Build history of the part. All positions in model axes, mm. A direction names the side the tool comes from. Give positions to 0.01 mm unless a question says otherwise; leave off trailing zeros. Write each loop counter-clockwise with the first axis right and the second up, starting at its lowest first coordinate (ties: lowest second). Pieces come first, ordered by that corner, then holes.
from build123d import *

# Parameters (mm, degrees)
SKETCH2_W           = 10
SKETCH2_H           = 10
BOSS_EXTRUDE1_DEPTH = 1.6
SKETCH4_W           = 10
SKETCH4_H           = 10
SKETCH4_W_2         = 7.6
SKETCH4_H_2         = 7.6
EXTRUDE_THIN1_DEPTH = 4
CUT_EXTRUDE1_DEPTH  = 5.6
SKETCH6_R           = 1.75
CUT_EXTRUDE2_DEPTH  = 5.6


with BuildPart() as part:
    # Sketch2 → Boss-Extrude1 (new body)
    with BuildSketch(Plane(origin=(0, 0, 0), x_dir=(1, 0, 0), z_dir=(0, 1, 0))):
        Rectangle(SKETCH2_W, SKETCH2_H)
    extrude(amount=BOSS_EXTRUDE1_DEPTH)

    # Sketch4 → Extrude-Thin1 (add)
    with BuildSketch(Plane(origin=(0, 1.6, 0), x_dir=(1, 0, 0), z_dir=(0, 1, 0))):
        Rectangle(SKETCH4_W, SKETCH4_H)
        Rectangle(SKETCH4_W_2, SKETCH4_H_2, mode=Mode.SUBTRACT)
    extrude(amount=EXTRUDE_THIN1_DEPTH)

    # Sketch5 → Cut-Extrude1 (cut)
    with BuildSketch(Plane.XZ):
        Polygon((-5, 5), (5, 5), (5, -5), align=None)
    extrude(amount=-CUT_EXTRUDE1_DEPTH, mode=Mode.SUBTRACT)

    # Sketch6 → Cut-Extrude2 (cut)
    with BuildSketch(Plane.XZ):
        with Locations((-5, -5)):
            Circle(SKETCH6_R)
    extrude(amount=-CUT_EXTRUDE2_DEPTH, mode=Mode.SUBTRACT)


solid = part.part
1. Saw through at D-D on x = 4. Give the cut face in (y, z), plus the area to 3 significant figures.
2. Saw through at C-C on x = 0.5. Give the cut face in (y, z), plus the area to 3 significant figures.
3. Saw through at A-A on y = 2.2. Give the cut face in (x, z), plus the area to 3 significant figures.
4. Drill centre lines: line 1 along X through (y, z) = (3.4, -1); line 2 along X through (y, z) = (1.2, -4.5). Where is each one in solid material? Low to high.
5. Drop flat-ended pins along their axis: pin 1 (1.2 mm diameter, centred on y = 4, z = 1.5, fed in from +X); pin 2 (2.5 mm diameter, centred on x = 0.5, z = 0.5, fed in from +Y); pin 3 (1 mm diameter, centred on x = 3.5, y = 2, fed in from +Z). Give the stop position or say it passes through.
6. 3-axis set-ups, long thin cutter, end or side, ignore diameter. For faces 1 (the face through (-1, 1.6, -1)), 2 (the face through (0, 4, -3.8)), 3 (the face through (-3.8, 4, 0)): which of +Z, -Z, +X, -X, +Y, -Y reach the whole face in a straight line?
7. Saw through at B-B on z = 2.5. Give the cut face in (x, y).
Outcome:
1. outline: (0, -5) - (5.6, -5) - (5.6, -4) - (0, -4) - close
1. area: 5.60 mm2
2. outline: (0, -5) - (5.6, -5) - (5.6, -3.8) - (1.6, -3.8) - (1.6, -0.5) - (0, -0.5) - close
2. area: 12.0 mm2
3. outline: (-5, -3.25) arc R1.75 cw to (-3.8, -3.73) - (-3.8, 3.8) - (-5, 5) - close; (-3.73, -3.8) arc R1.75 cw to (-3.25, -5) - (5, -5) - (3.8, -3.8) - close
3. area: 18.7 mm2
4. line 1: x = -5 to -3.8
4. line 2: x = -3.32 to 4.5
5. pin 1: stops at x = -3.8
5. pin 2: stops at y = 1.6
5. pin 3: stops at z = -3.2
6. face 1: +Z, +X, +Y
6. face 2: +Z, +X, -X, +Y
6. face 3: +Z, -Z, +X, +Y
7. outline: (-5, 0) - (-2.5, 0) - (-2.5, 1.6) - (-3.8, 1.6) - (-3.8, 5.6) - (-5, 5.6) - close
